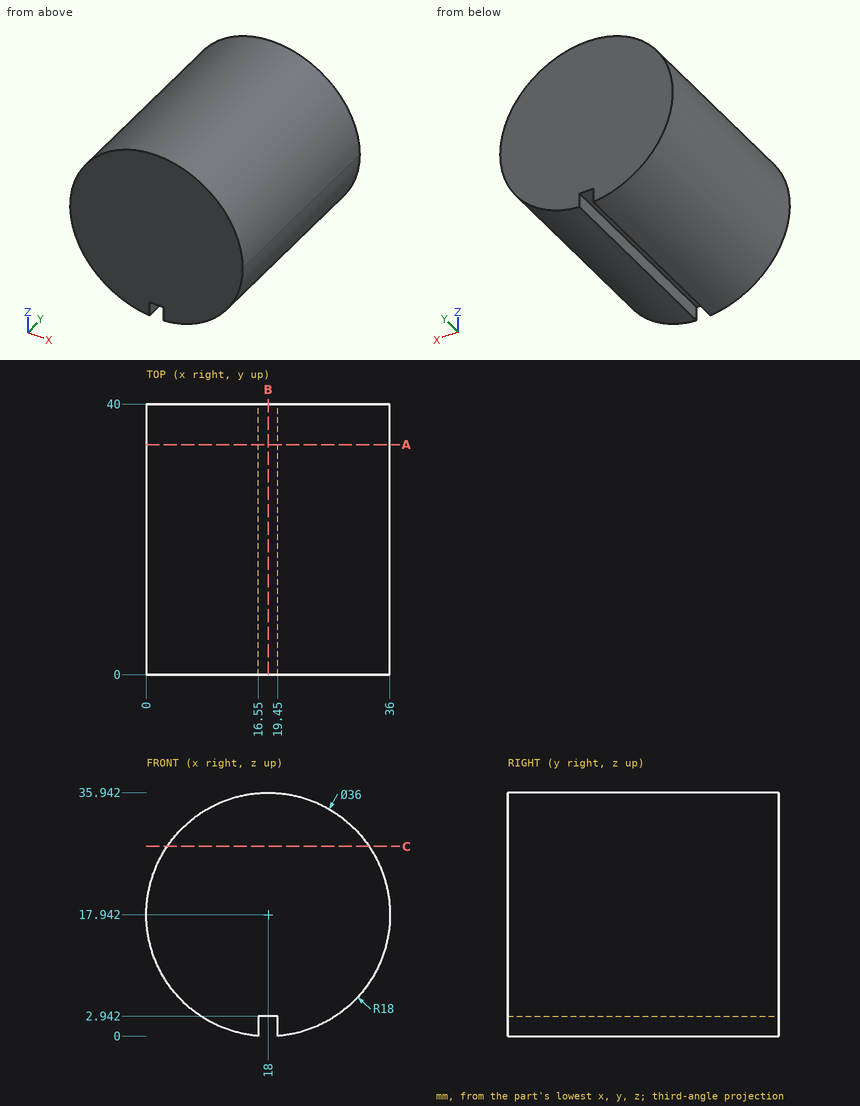
Answer from the drawing. Dimensions are ordinates in mm from the lowest x, y and z of the part. Coordinates: 2 decimals unless noted, no trailing zeros. Loops run counter-clockwise (first coordinate to the right, second up) from the corner with the lowest first, then second, coordinate; pieces in that order, holes last.
Q1. The part is cut by section C-C on z = 28. Write down the section's boundary in (x, y), and give its area (3 significant figures).
Q2. The part is cut by section A-A on y = 34. Write down the section's boundary in (x, z), and give its area (3 significant figures).
Q3. Each of these flat-tipped pins is pushed along its axis until it touches: pin 1 Ø4 at (y, z) = (9, 10) entering from +X; pin 2 Ø1.5 at (y, z) = (28, 2) entering from -X (1 decimal); pin 3 Ø10 at (x, y) = (27.5, 32.5) entering from +Z. Where does it stop, or does it pass through?
Q4. The part is cut by section B-B on x = 18. Write down the section's boundary in (y, z).
Q5. Consider probe 1 along X at (y, z) = (20, 25.5) (1 decimal); probe 2 along Z at (x, y) = (10, 7) (1 decimal); probe 3 along X at (y, z) = (20, 17.5) (1 decimal). Determine where each line is inside the solid, lowest interval first.
Results below:
1. outline: (3.07, 0) - (32.93, 0) - (32.93, 40) - (3.07, 40) - close
1. area: 1,190 mm2
2. outline: (16.55, 0) - (16.55, 2.94) - (19.45, 2.94) - (19.45, 0) arc R18 ccw (long way) to start
2. area: 1,010 mm2
3. pin 1: stops at x = 34.99
3. pin 2: stops at x = 8.3
3. pin 3: stops at z = 35.37
4. outline: (0, 2.94) - (40, 2.94) - (40, 35.94) - (0, 35.94) - close
5. probe 1: x = 1.7 to 34.3
5. probe 2: z = 1.8 to 34.1
5. probe 3: x = 0 to 36
